Build history of the part. All positions in model axes, mm. Face numbers are marked on the shaded views. A direction names the side the tool comes from. Give positions to 0.01 mm unless a question says otherwise; leave off trailing zeros. Write each loop counter-clockwise with the first axis right and the second up, starting at its lowest first coordinate (ties: lowest second). Pieces come first, ordered by that corner, then holes. Notation, with made-up numbers: (-16, 6) -> (5, 6) arc R18 cw to (5, 14) -> close; hole circle Ø9 at (51, 86.5). An arc over 180 degrees is marked (long way). Put each result on its own line as item: value.
Autodesk Inventor part; units mm, degrees
ref_plane "YZ Plane" through (0, 0, 0) normal (1, 0, 0) x (0, 1, 0)
ref_plane "XZ Plane" through (0, 0, 0) normal (0, 1, 0) x (-1, 0, 0)
ref_plane "XY Plane" through (0, 0, 0) normal (0, 0, 1) x (1, 0, 0)
sketch "Sketch1" plane through (0, 0, 0) normal (1, 0, 0) x (0, 1, 0)
  line L0 (4, -10.5) -> (4, 0)
  line L1 (0, 0) -> (0, -10.5)
  line L2 (4, -10.5) -> (5, -10.5)
  line L3 (5, -10.5) -> (5, -9)
  line L4 (5, -9) -> (11, -9)
  line L5 (11, -9) -> (11, -5.5)
  line L6 (11, -5.5) -> (5, -5.5)
  line L7 (5, -5.5) -> (5, 0)
  line L8 (5, 0) -> (4, 0)
  dimension "d0" = 10.5
  dimension "d1" = 4
  dimension "d2" = 5
  dimension "d3" = 5
  dimension "d4" = 3.5
  dimension "d10" = 11
revolve "Revolution1" add sketch "Sketch1" angle 360 about axis through (0, 0, 0) along (0, 0, -1)
sketch "Sketch2" plane through (0, 0, -5.5) normal (0, 0, 1) x (1, 0, 0)
  point P0 (0, 0)
  point P1 (0, 7.75)
  point P2 (-7.75, 0)
  point P3 (0, -7.75)
  point P4 (7.75, 0)
  dimension "d6" = 15.5
  dimension "d7" = 7.75
  dimension "d8" = 15.5
  dimension "d9" = 7.75
hole "Hole1" at (0, 7.75, -5.5) at (-7.75, 0, -5.5) at (0, -7.75, -5.5) at (7.75, 0, -5.5) direction (0, 0, -1) diameter 2.459 end through all
properties part number "Z Axis Nut" material "Brass, Soft Yellow"
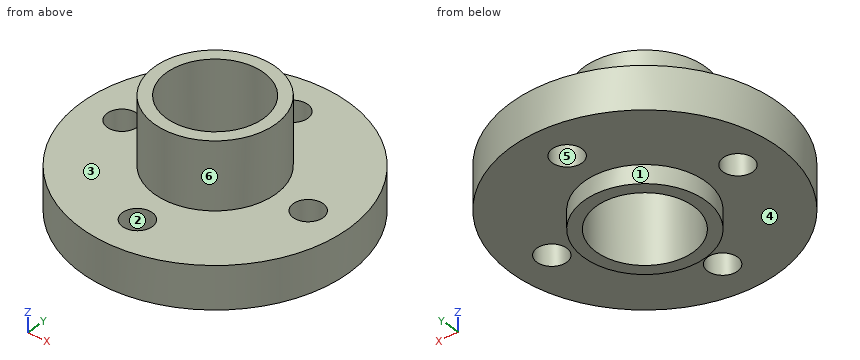
1) Slice it at C-C (y = 7.75). Write the cut outline in (x, z), plus the area to 3 significant figures.
Filled sheet:
outline: (-7.81, -9) -> (-1.23, -9) -> (-1.23, -5.5) -> (-7.81, -5.5) -> close; (1.23, -9) -> (7.81, -9) -> (7.81, -5.5) -> (1.23, -5.5) -> close
area: 46.0 mm2
2) Slice it at B-B (z = -6.25). Write the cut outline in (x, y).
Filled sheet:
outline: circle Ø22 at (0, 0); hole circle Ø2.46 at (-7.75, 0); hole circle Ø8 at (0, 0); hole circle Ø2.46 at (0, -7.75); hole circle Ø2.46 at (0, 7.75); hole circle Ø2.46 at (7.75, 0)
3) Tool access for the marked faces 1, 2 and 3: list every direction of +Z, -Z, +X, -X, +Y, -Y with a clear straight run to the whole face (end or side of a thin tool).
Filled sheet:
face 1: -Z
face 2: +Z, -Z
face 3: +Z
4) Pin check, flat tips, straight feed: pin 1 (1 mm diameter, centred on x = 6, y = 2.5, fed in from -Z); pin 2 (3 mm diameter, centred on x = -7.75, y = 0, fed in from +Z); pin 3 (3 mm diameter, centred on x = -3.5, z = -9, fed in from +Y). Stop position of each tip, or through.
Filled sheet:
pin 1: z = -9
pin 2: z = -5.5
pin 3: y = 10.82
5) Pull direction X, two halves, no side cores. Call the marked faces 4, 5 and 6: released by +X, released by -X, zero draft, split by the parting line, or undercut.
Filled sheet:
face 4: zero draft
face 5: undercut
face 6: split by the parting line
6) Wall check: L1, parallel to X at y = 0, z = -6.5; L2, parallel to Z at x = 1.75, y = 8; L3, parallel to Y at x = 7.75, z = -7.65. Give the ranges that are in metal, low to high.
Filled sheet:
L1: -11 to -8.98, -6.52 to -4, 4 to 6.52, 8.98 to 11
L2: -9 to -5.5
L3: -7.81 to -1.23, 1.23 to 7.81
7) Slice it at A-A (x = 0). Write the cut outline in (y, z).
Filled sheet:
outline: (-11, -9) -> (-8.98, -9) -> (-8.98, -5.5) -> (-11, -5.5) -> close; (-6.52, -9) -> (-5, -9) -> (-5, -10.5) -> (-4, -10.5) -> (-4, 0) -> (-5, 0) -> (-5, -5.5) -> (-6.52, -5.5) -> close; (4, -10.5) -> (5, -10.5) -> (5, -9) -> (6.52, -9) -> (6.52, -5.5) -> (5, -5.5) -> (5, 0) -> (4, 0) -> close; (8.98, -9) -> (11, -9) -> (11, -5.5) -> (8.98, -5.5) -> close
